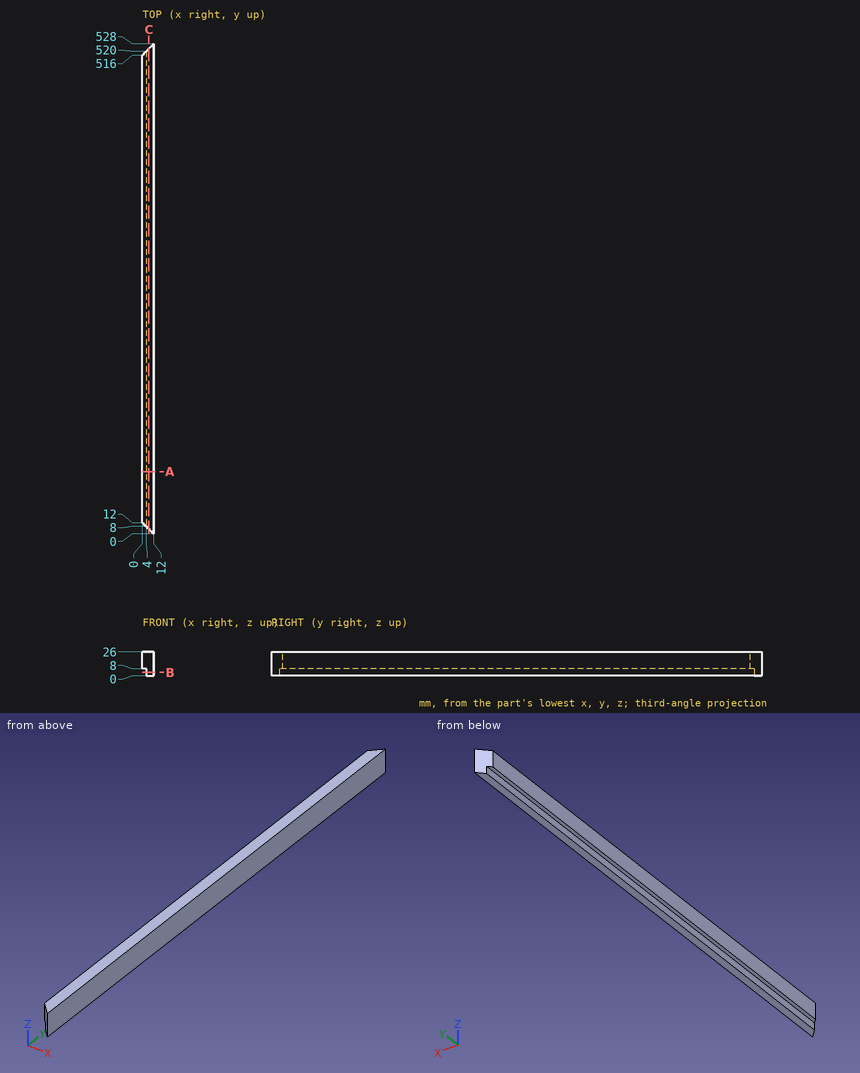
Could you check a few things on this drawing? It's one solid part, dimensions in mm from its lowest x, y, z. Round coordinates to 2 decimals unless told otherwise and drop trailing zeros. Order: outer loops, then holes, each group sorted by start corner. A loop starts at its lowest first (then second) coordinate and runs counter-clockwise, first axis right, second up.
(1) Imagine slicing it at B-B (z = 4). Write out the boundary of the cut face in (x, y).
Response values:
outline: (4, 8) - (12, 0) - (12, 528) - (4, 520) - close
(2) Imagine slicing it at C-C (x = 7). Write out the boundary of the cut face in (y, z), plus the area to 3 significant figures.
Response values:
outline: (5, 0) - (523, 0) - (523, 26) - (5, 26) - close
area: 13,500 mm2
(3) Please list where these lines run through material, in increasing order: line 1 along Z through (x, y) = (3.5, 214); line 2 along X through (y, z) = (455.5, 5); line 3 along Y through (x, z) = (4.5, 19.5).
Response values:
line 1: z = 8 to 26
line 2: x = 4 to 12
line 3: y = 7.5 to 520.5
(4) I'm going to push flat-ended pins straight in: pin 1 (6.5 mm diameter, centred on y = 225, z = 3.5, fed in from -X); pin 2 (6 mm diameter, centred on x = 8, z = 18, fed in from -Y); pin 3 (3 mm diameter, centred on x = 9, z = 10.5, fed in from +Y). Where does each tip first touch, or does it pass through?
Response values:
pin 1: stops at x = 4
pin 2: stops at y = 1
pin 3: stops at y = 526.5
(5) Imagine slicing it at A-A (y = 67). Write out the boundary of the cut face in (x, z).
Response values:
outline: (0, 8) - (4, 8) - (4, 0) - (12, 0) - (12, 26) - (0, 26) - close
